```python
from build123d import *

# Parameters (mm, degrees)
BOSS_EXTRUDE1_DEPTH      = 150
BOSS_EXTRUDE1_DEPTH_BACK = 5
SKETCH1_W                = 180
SKETCH1_H                = 180
SKETCH6_W                = 175
SKETCH6_H                = 175
CUT_EXTRUDE2_DEPTH       = 150
SKETCH34_W               = 180
SKETCH34_H               = 180
BOSS_EXTRUDE14_DEPTH     = 5
SKETCH35_W               = 15.2
SKETCH35_H               = 15.2
CUT_EXTRUDE11_DEPTH      = 5
SKETCH37_W               = 14.2
SKETCH37_H               = 14.2
CUT_EXTRUDE12_DEPTH      = 5
MIRROR13_COPY_1_SKETCH_W = 15.2
MIRROR13_COPY_1_SKETCH_H = 15.2
MIRROR13_COPY_1_DEPTH    = 5
MIRROR13_COPY_2_SKETCH_W = 14.2
MIRROR13_COPY_2_SKETCH_H = 14.2
MIRROR13_COPY_2_DEPTH    = 5
SKETCH15_W               = 10
SKETCH15_H               = 10
CUT_EXTRUDE7_DEPTH       = 3
SKETCH21_W               = 50
SKETCH21_H               = 3
BOSS_EXTRUDE7_DEPTH      = 10
SKETCH22_W               = 2.5
SKETCH22_H               = 10
BOSS_EXTRUDE8_DEPTH      = 5
SKETCH30_W               = 45
SKETCH30_H               = 2.5
CUT_EXTRUDE9_DEPTH       = 5
SKETCH38_W               = 70.2
SKETCH38_H               = 70.2
CUT_EXTRUDE13_DEPTH      = 5
SKETCH7_R                = 25.65
CUT_EXTRUDE14_DEPTH      = 5
CUT_EXTRUDE16_START      = -1.5
SKETCH39_R               = 27.15
CUT_EXTRUDE16_DEPTH      = 2


with BuildPart() as part:
    # Sketch1 → Boss-Extrude1 (new, two sides: drawn at the far end of the back side and taken through both)
    with BuildSketch(Plane(origin=(0, 0, 0), x_dir=(1, 0, 0), z_dir=(0, 1, 0)).offset(-BOSS_EXTRUDE1_DEPTH_BACK)):
        Rectangle(SKETCH1_W, SKETCH1_H)
    extrude(amount=BOSS_EXTRUDE1_DEPTH + BOSS_EXTRUDE1_DEPTH_BACK)

    # Sketch6 → Cut-Extrude2 (cut)
    with BuildSketch(Plane(origin=(0, 150, 0), x_dir=(1, 0, 0), z_dir=(0, 1, 0))):
        Rectangle(SKETCH6_W, SKETCH6_H)
    extrude(amount=-CUT_EXTRUDE2_DEPTH, mode=Mode.SUBTRACT)

    # Sketch34 → Boss-Extrude14 (add)
    with BuildSketch(Plane.XZ.offset(5)):
        Rectangle(SKETCH34_W, SKETCH34_H)
    extrude(amount=BOSS_EXTRUDE14_DEPTH)

    # Sketch35 → Cut-Extrude11 (cut)
    with BuildSketch(Plane.XZ.offset(10)):
        with Locations((-75.5, 75.5)):
            Rectangle(SKETCH35_W, SKETCH35_H)
    cut_extrude11 = extrude(amount=-CUT_EXTRUDE11_DEPTH, mode=Mode.SUBTRACT)

    # Sketch37 → Cut-Extrude12 (cut)
    with BuildSketch(Plane(origin=(0, 0, 0), x_dir=(1, 0, 0), z_dir=(0, 1, 0))):
        with Locations((-55.5, -33.75)):
            Rectangle(SKETCH37_W, SKETCH37_H)
    cut_extrude12 = extrude(amount=-CUT_EXTRUDE12_DEPTH, mode=Mode.SUBTRACT)

    # Mirror12: Cut-Extrude11, Cut-Extrude12 across plane
    add(cut_extrude11.mirror(Plane.XY), mode=Mode.SUBTRACT)
    add(cut_extrude12.mirror(Plane.XY), mode=Mode.SUBTRACT)

    # Mirror13: Cut-Extrude11, Cut-Extrude12 across plane
    add(cut_extrude11.mirror(Plane(origin=(0, 0, 0), x_dir=(0, 0, 1), z_dir=(1, 0, 0))), mode=Mode.SUBTRACT)
    add(cut_extrude12.mirror(Plane(origin=(0, 0, 0), x_dir=(0, 0, 1), z_dir=(1, 0, 0))), mode=Mode.SUBTRACT)

    # Mirror13 copy 1 sketch → Mirror13 copy 1 (cut)
    with BuildSketch(Plane(origin=(0, -10, 0), x_dir=(-1, 0, 0), z_dir=(0, -1, 0))):
        with Locations((-75.5, 75.5)):
            Rectangle(MIRROR13_COPY_1_SKETCH_W, MIRROR13_COPY_1_SKETCH_H)
    extrude(amount=-MIRROR13_COPY_1_DEPTH, mode=Mode.SUBTRACT)

    # Mirror13 copy 2 sketch → Mirror13 copy 2 (cut)
    with BuildSketch(Plane(origin=(0, 0, 0), x_dir=(-1, 0, 0), z_dir=(0, 1, 0))):
        with Locations((-55.5, -33.75)):
            Rectangle(MIRROR13_COPY_2_SKETCH_W, MIRROR13_COPY_2_SKETCH_H)
    extrude(amount=-MIRROR13_COPY_2_DEPTH, mode=Mode.SUBTRACT)

    # Sketch15 → Cut-Extrude7 (cut)
    with BuildSketch(Plane(origin=(90, 0, 0), x_dir=(0, 0, -1), z_dir=(1, 0, 0))):
        with Locations((0.004832502, 145)):
            Rectangle(SKETCH15_W, SKETCH15_H)
    cut_extrude7 = extrude(amount=-CUT_EXTRUDE7_DEPTH, mode=Mode.SUBTRACT)

    # Mirror3: Cut-Extrude7 across plane
    add(cut_extrude7.mirror(Plane(origin=(0, 0, 0), x_dir=(0, 0, 1), z_dir=(1, 0, 0))), mode=Mode.SUBTRACT)

    # Sketch21 → Boss-Extrude7 (add)
    with BuildSketch(Plane(origin=(0, 0, 87.5), x_dir=(-1, 0, 0), z_dir=(0, 0, -1))):
        with Locations((0.003304144, 88.502007714)):
            Rectangle(SKETCH21_W, SKETCH21_H)
    extrude(amount=BOSS_EXTRUDE7_DEPTH)

    # Sketch22 → Boss-Extrude8 (add)
    with BuildSketch(Plane(origin=(0, 90.002007714, 0), x_dir=(1, 0, 0), z_dir=(0, 1, 0))):
        with Locations((-23.753304144, -82.5)):
            Rectangle(SKETCH22_W, SKETCH22_H)
    boss_extrude8 = extrude(amount=BOSS_EXTRUDE8_DEPTH)

    # Mirror7: Boss-Extrude8 across plane
    add(boss_extrude8.mirror(Plane(origin=(0, 0, 0), x_dir=(0, 0, 1), z_dir=(1, 0, 0))))

    # Sketch30 → Cut-Extrude9 (cut)
    with BuildSketch(Plane(origin=(0, 150, 0), x_dir=(1, 0, 0), z_dir=(0, 1, 0))):
        with Locations((0.002512985, 88.75)):
            Rectangle(SKETCH30_W, SKETCH30_H)
    extrude(amount=-CUT_EXTRUDE9_DEPTH, mode=Mode.SUBTRACT)

    # Sketch38 → Cut-Extrude13 (cut)
    with BuildSketch(Plane(origin=(0, 0, 0), x_dir=(1, 0, 0), z_dir=(0, 1, 0))):
        Rectangle(SKETCH38_W, SKETCH38_H)
    extrude(amount=-CUT_EXTRUDE13_DEPTH, mode=Mode.SUBTRACT)

    # Sketch7 → Cut-Extrude14 (cut)
    with BuildSketch(Plane(origin=(0, -5, 0), x_dir=(1, 0, 0), z_dir=(0, 1, 0))):
        with Locations(Location((0, 0, 0), (0, 0, 270))):
            Circle(SKETCH7_R)
    extrude(amount=-CUT_EXTRUDE14_DEPTH, mode=Mode.SUBTRACT)

    # Sketch39 → Cut-Extrude16 (cut)
    with BuildSketch(Plane(origin=(0, -5, 0), x_dir=(1, 0, 0), z_dir=(0, 1, 0)).offset(CUT_EXTRUDE16_START)):
        with Locations(Location((0, 0, 0), (0, 0, 270))):
            Circle(SKETCH39_R)
    extrude(amount=-CUT_EXTRUDE16_DEPTH, mode=Mode.SUBTRACT)


solid = part.part
```
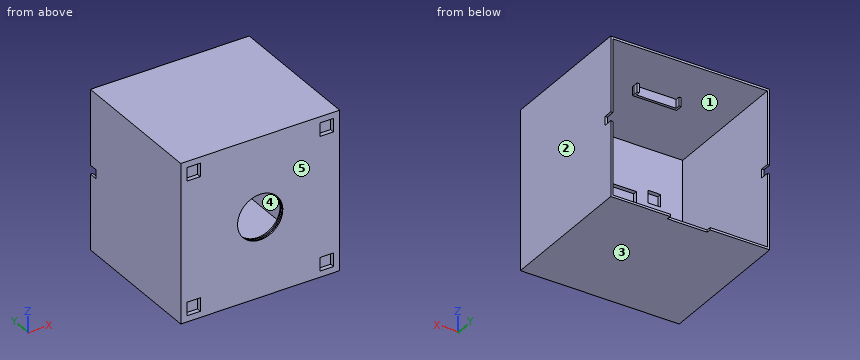
Here's how the part is built. I have some questions about the finished solid (model axes, mm). Face numbers are marked on the shaded views. A direction names the side the tool comes from. Coordinates: 2 decimals unless noted, no trailing zeros. Loops run counter-clockwise (first coordinate to the right, second up) from the corner with the lowest first, then second, coordinate; pieces in that order, holes last. Notation, with made-up numbers: (-9, 19) -> (1, 19) arc R26 ccw to (1, 33) -> close; hole circle Ø9 at (-34.5, -20.75). An arc over 180 degrees is marked (long way). Return JSON: item names as keys, results as strings.
1) I need wall thicknesses on line 1 (Z direction, x = 41.5, y = 30.5); line 2 (X direction, y = -6, z = 0). Which ranges of each line are inside material? Lowest first, please. Write a range as from..to.
Results below:
{"line 1": "-90..-87.5, 87.5..90", "line 2": "-90..-25.65, 25.65..90"}
2) For the marked faces 4 and 5, which set-ups out of +Z, -Z, +X, -X, +Y, -Y let a thin tool reach every point of the face, with its end or its side?
Results below:
{"face 4": "+Y", "face 5": "+Z, -Z, +X, -X, -Y"}
3) Thinking about a two-plate mould opening in X: for the marked faces 1, 2 and 3, which applies, +X half, -X half, draft (parallel to the pull), parting line (faces both ways), or undercut?
Results below:
{"face 1": "undercut", "face 2": "+X half", "face 3": "draft"}
4) If we section it at C-C, the plane y = 104: Write out the boundary of the cut face in (x, z).
Results below:
{"outline": "(-90, -90) -> (90, -90) -> (90, 90) -> (-90, 90) -> close; hole (-87.5, -87.5) -> (87.5, -87.5) -> (87.5, 87.5) -> (-87.5, 87.5) -> close"}
5) If we section it at A-A, the plane z = 0: Write out the boundary of the cut face in (x, y).
Results below:
{"outline": "(-90, -10) -> (-25.65, -10) -> (-25.65, -8.5) -> (-27.15, -8.5) -> (-27.15, -6.5) -> (-25.65, -6.5) -> (-25.65, -5) -> (-35.1, -5) -> (-35.1, 0) -> (-87.5, 0) -> (-87.5, 140) -> (-90, 140) -> close; (25.65, -10) -> (90, -10) -> (90, 140) -> (87.5, 140) -> (87.5, 0) -> (35.1, 0) -> (35.1, -5) -> (25.65, -5) -> (25.65, -6.5) -> (27.15, -6.5) -> (27.15, -8.5) -> (25.65, -8.5) -> close"}
6) Will these pins go through, and if not, where does the flat tip stop? pin 1 (4.5 mm diameter, centred on x = 54.5, z = -36, fed in from +Y); pin 2 (1.2 mm diameter, centred on x = 89, z = 2, fed in from +Y); pin 3 (12 mm diameter, centred on x = 47, z = -6.5, fed in from +Y).
Results below:
{"pin 1": "y = -5", "pin 2": "y = 140", "pin 3": "y = 0"}
7) If we section it at B-B, the plane x = 0: Write out the boundary of the cut face in (y, z).
Results below:
{"outline": "(-10, -90) -> (145, -90) -> (145, -87.5) -> (0, -87.5) -> (0, -35.1) -> (-5, -35.1) -> (-5, -25.65) -> (-6.5, -25.65) -> (-6.5, -27.15) -> (-8.5, -27.15) -> (-8.5, -25.65) -> (-10, -25.65) -> close; (-10, 25.65) -> (-8.5, 25.65) -> (-8.5, 27.15) -> (-6.5, 27.15) -> (-6.5, 25.65) -> (-5, 25.65) -> (-5, 35.1) -> (0, 35.1) -> (0, 87.5) -> (87, 87.5) -> (87, 77.5) -> (90, 77.5) -> (90, 87.5) -> (150, 87.5) -> (150, 90) -> (-10, 90) -> close"}
8) If we section it at D-D, the plane z = 50.5: Write out the boundary of the cut face in (x, y).
Results below:
{"outline": "(-90, -10) -> (90, -10) -> (90, 150) -> (87.5, 150) -> (87.5, 0) -> (-87.5, 0) -> (-87.5, 150) -> (-90, 150) -> close"}
